```python
from build123d import *

# Parameters (mm, degrees)
F0_W     = 19.05
F0_H     = 19.05
F0_W_2   = 12.7
F0_H_2   = 12.7
F1_DEPTH = 508
F2_R     = 3.175
F3_DEPTH = 63.5


with BuildPart() as f1:
    # F0 (on Front) → F1 (new body)
    with BuildSketch(Plane.XZ):
        with Locations((-6.35, 6.35)):
            Rectangle(F0_W, F0_H)
        with Locations((-6.35, 6.35)):
            Rectangle(F0_W_2, F0_H_2, mode=Mode.SUBTRACT)
    extrude(amount=F1_DEPTH)

    # F2 (on Top) → F3 (cut, symmetric)
    with BuildSketch(Plane.XY):
        with Locations((-6.35, -12.7)):
            Circle(F2_R)
        with Locations((-6.35, -254)):
            Circle(F2_R)
        with Locations((-6.35, -495.3)):
            Circle(F2_R)
    extrude(amount=F3_DEPTH, both=True, mode=Mode.SUBTRACT)


solid = f1.part
```
Geometry: final body of the model. Coordinates: model frame, mm. A direction names the side the tool comes from. Round coordinates to 2 decimals unless told otherwise and drop trailing zeros. Write each loop counter-clockwise with the first axis right and the second up, starting at its lowest first coordinate (ties: lowest second). Pieces come first, ordered by that corner, then holes. Notation, with made-up numbers: (28, 2.25) -> (63, 2.25) arc R26 cw to (63, 16.25) -> close; hole circle Ø7 at (-7, 0). An arc over 180 degrees is marked (long way). Use CSV: the item, a comma, the result in double quotes. Start each with the question number.
Q1. Section B-B (x = -6.35). Give the number of separate pieces and of enclosed holes in the cut face, plus the area to 3 significant figures.
Q2. Reachability of faces 1 (the face through (-12.7, -250, 6)), 2 (the face through (3.175, -250, 6)) from +Z, -Z, +X, -X, +Y, -Y: full face, straight path, thin tool, end or side. Return the list, or none.
Q3. Section A-A (z = 9). Return loops of the section in (x, y) (3 decimals).
Q4. Line query: L1, parallel to Y at x = -6.35, z = -0.85 (3 decimals); L2, parallel to Z at x = -12, y = -419.5 (3 decimals); L3, parallel to X at y = -254, z = -1.3 (3 decimals). Output: solid intervals per line, ascending.
Q5. Pull-direction query (Z, two-part tool) for faces 3 (the face through (-15.875, -250, 6)), 4 (the face through (-6, -250, 12.7)), 5 (the face through (-6, -250, 15.875)); classes: pulls with the +Z half, pulls with the -Z half, needs draft (parallel to the pull), parting line crosses it, or undercut.
Q6. Section C-C (y = -31). Return loops of the section in (x, z) (3 decimals), plus the area to 3 significant figures.
Result sheet:
1,separate pieces,"8"
1,enclosed holes,"0"
1,area,"3,100 mm²"
2,face 1,"+Y, -Y"
2,face 2,"+Z, -Z, +X, +Y, -Y"
3,outline,"(-15.875, -508) -> (-12.7, -508) -> (-12.7, 0) -> (-15.875, 0) -> close; (0, -508) -> (3.175, -508) -> (3.175, 0) -> (0, 0) -> close"
4,L1,"-508 to -498.475, -492.125 to -257.175, -250.825 to -15.875, -9.525 to 0"
4,L2,"-3.175 to 0, 12.7 to 15.875"
4,L3,"-15.875 to -9.525, -3.175 to 3.175"
5,face 3,"needs draft"
5,face 4,"undercut"
5,face 5,"pulls with the +Z half"
6,outline,"(-15.875, -3.175) -> (3.175, -3.175) -> (3.175, 15.875) -> (-15.875, 15.875) -> close; hole (-12.7, 0) -> (0, 0) -> (0, 12.7) -> (-12.7, 12.7) -> close"
6,area,"202 mm²"
